The model under review builds one solid part; all positions refer to its coordinate system, in mm. Face numbers are marked on the shaded views. A direction names the side the tool comes from. Give positions to 0.01 mm unless a question says otherwise; leave off trailing zeros. Write each question's results on one line, items separated by ' | '. Start each with the question number.
from build123d import *

# Parameters (mm, degrees)
SKETCH17_R         = 4.826
CUT_EXTRUDE3_DEPTH = 12.7
SKETCH19_R         = 8.255
CUT_EXTRUDE4_DEPTH = 10.16
CIRPATTERN1_COUNT  = 3


with BuildPart() as part:
    # Sketch16 → Revolve5 (revolve)
    with BuildSketch(Plane.XY):
        with BuildLine():
            Line((0, 0), (38.1, 0))
            Line((38.1, 0), (38.1, 19.812))
            add(Edge.make_bspline(
                [(0, 0), (0, 21.471640273), (38.1, 19.812)],
                knots=[0, 0, 0, 1, 1, 1], degree=2))
        make_face()
    revolve(axis=Axis((0, 0, 0), (1, 0, 0)))

    # Sketch17 → Cut-Extrude3 (cut)
    with BuildSketch(Plane(origin=(38.1, 0, 0), x_dir=(0, 0, -1), z_dir=(1, 0, 0))):
        Circle(SKETCH17_R)
    extrude(amount=-CUT_EXTRUDE3_DEPTH, mode=Mode.SUBTRACT)

    # Sketch19 → Cut-Extrude4 (cut, symmetric)
    with BuildSketch(Plane(origin=(0, 19.812, 0), x_dir=(1, 0, 0), z_dir=(0, 1, 0))):
        with Locations(Location((25.4, 0, 0), (0, 0, 270))):
            Circle(SKETCH19_R)
    cut_extrude4 = extrude(amount=CUT_EXTRUDE4_DEPTH, both=True, mode=Mode.SUBTRACT)

    # CirPattern1: Cut-Extrude4 ×3 about axis
    cirpattern1_axis = Axis((0, 0, 0), (1, 0, 0))
    for i in range(1, CIRPATTERN1_COUNT):
        add(cut_extrude4.rotate(cirpattern1_axis, i * 360 / CIRPATTERN1_COUNT), mode=Mode.SUBTRACT)


solid = part.part
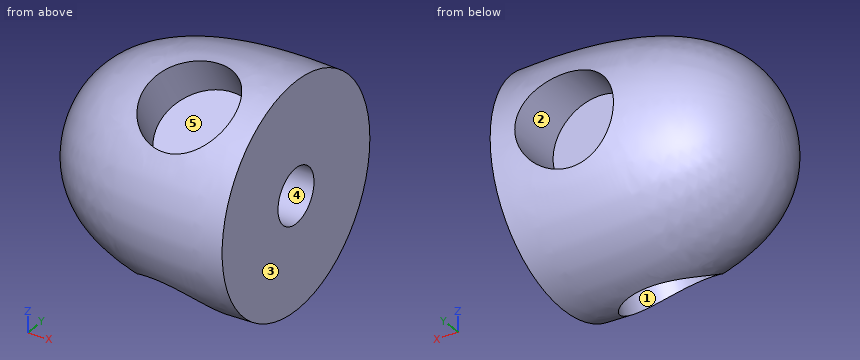
(1) Draft analysis for pull direction X (two halves, no side actions). For the marked faces 3, 4 and 5, state which applies: pulls with the +X half, pulls with the -X half, needs draft (parallel to the pull), parting line crosses it, or undercut.
(2) Add section A-A (y = 0). Give the number of separate pieces and of enclosed holes in the cut face, then the cut area to 3 significant figures.
(3) Wall thickness on L1, parallel to Y at x = 28.5, z = 0; L2, parallel to X at y = -13, z = -8.5; L3, parallel to Y at x = 30.5, z = 0: over which ranges is each line inside the solid? List them lowest first.
(4) Clearance check with flat-ended pins moving along their axes: P1, Ø5, axis at y = 15.5, z = -7, coming from the -X side; P2, Ø10, axis at x = 20, y = -8, coming from the +Z side; P3, Ø10, axis at y = -5.5, z = -14.5, coming from the -X side; P4, Ø10.5, axis at y = -1.5, z = 1, coming from the +X side. State where each tip first meets the part, or that it passes through.
(5) Machinability: for the marked faces 1 and 2, which of the approach directions +Z, -Z, +X, -X, +Y, -Y give a long, thin tool a straight path to every point of the face, cutting with its end or side? Answer none if there is none.
Calculated:
1) face 3: pulls with the +X half | face 4: needs draft | face 5: undercut
2) separate pieces: 1 | enclosed holes: 2 | area: 1,090 mm²
3) L1: y = -19.84 to -4.83, 4.83 to 9.65 | L2: x = 9.23 to 21.04, 29.76 to 38.1 | L3: y = -19.91 to -4.83, 4.83 to 9.65
4) P1: stops at x = 7.51 | P2: stops at z = 18.84 | P3: stops at x = 3.2 | P4: stops at x = 38.1
5) face 1: none | face 2: +Y
